Read the model definition and answer for the solid it produces. Units are mm, in the model's axes. A direction names the side the tool comes from. Give positions to 0.01 mm unless a question says otherwise; leave off trailing zeros. Write each loop counter-clockwise with the first axis right and the second up, starting at its lowest first coordinate (ties: lowest second). Pieces come first, ordered by that corner, then holes. Notation, with made-up numbers: (43, -1.5) -> (97, -1.5) arc R14 ccw to (97, 4.5) -> close; hole circle Ø8 at (-32.5, -28). An arc over 180 degrees is marked (long way). Put each result on its own line as item: value. Start each with the question number.
from build123d import *

# Parameters (mm, degrees)
PAD002_DEPTH = 12
PAD_DEPTH    = 2
ARRAY_COUNT  = 3


with BuildPart() as pad002:
    # Sketch002 → Pad002 (new body)
    with BuildSketch(Plane.XY):
        Polygon((-6.6395280957, 11.5), (-7.7942286341, 13.5), (-68, 13.5), (-68, -13.5), (-7.7942286341, -13.5), (-6.6395280957, -11.5), (-66, -11.5), (-66, 11.5), align=None)
    extrude(amount=PAD002_DEPTH)


with BuildPart() as array:
    # Sketch → Pad (new body)
    with BuildSketch(Plane.XY):
        Polygon((0, 0), (-7.7942286341, 13.5), (-68, 13.5), (-68, -13.5), (-7.7942286341, -13.5), align=None)
    extrude(amount=PAD_DEPTH)

    # Fusion: union Pad002
    add(pad002.part)

    # Array: Array ×3 about axis
    array_axis = Axis((0, 0, 0), (0, 0, 1))


with BuildPart() as array_1:
    add(array.part)
    for i in range(1, ARRAY_COUNT):
        add(array.part.rotate(array_axis, i * 360 / ARRAY_COUNT))


solid = array_1.part
1) Straight lines are drawn through the part: line 1 (Y direction, x = 16, z = 8.25); line 2 (Y direction, x = -28, z = 9.25); line 3 (Z direction, x = -63, y = 5). For each, find the intervals that lie inside material, in ascending order. Write a range as [from, to].
2) For faces 4 (the face through (30.429, 25.705, 5.916)), 5 (the face through (0, -1, 0)), 6 (the face through (-37, 11.5, 7)), 7 (the face through (-37, 13.5, 6)), 8 (the face through (-38, -13.5, 6)), determine the directions among +Z, -Z, +X, -X, +Y, -Y from which every point of the face is accessible in a straight line to the end or side of a thin tool.
3) For a pull along Y with two mould halves and no side action, classify faces 1 (the face through (7.468, 39.935, 5.916)), 2 (the face through (-7, -12, 12)), 3 (the face through (-36, -11.5, 7)) as pulls with the +Y half, pulls with the -Y half, needs draft (parallel to the pull), parting line crosses it, or undercut.
4) A cutting plane is placed at C-C on y = -54. Give the vertices of the cut face in (x, z), and give its area (3 significant figures).
5) A cutting plane is placed at A-A on z = 3.5. Give the vertices of the cut face in (x, y).
6) Each of these flat-tipped pins is pushed along its axis until it touches: pin 1 Ø6 at (x, z) = (22, 7) entering from +Y; pin 2 Ø3 at (x, z) = (-49, 8) entering from -Y; pin 3 Ø4 at (y, z) = (-48.5, 5) entering from +X. Where does it stop, or does it pass through?
7) A cutting plane is placed at D-D on x = -21. Give the vertices of the cut face in (y, z), and give its area (3 significant figures).
8) A cutting plane is placed at B-B on x = 38. Give the vertices of the cut face in (y, z), and give its area (3 significant figures).
Results found:
1. line 1: y = [-54.71, -50.71], [-4.71, -0.71], [0.71, 4.71], [50.71, 54.71]
1. line 2: y = [-13.5, -11.5], [11.5, 13.5]
1. line 3: z = [0, 2]
2. face 4: +Z, -Z, +X
2. face 5: -Z, +X, -X, +Y, -Y
2. face 6: +Z
2. face 7: +Z, -Z, -X, +Y
2. face 8: +Z, -Z, -X, -Y
3. face 1: pulls with the +Y half
3. face 2: needs draft
3. face 3: undercut
4. outline: (15.59, 0) -> (42.47, 0) -> (42.47, 12) -> (38.47, 12) -> (38.47, 2) -> (17.9, 2) -> (17.9, 12) -> (15.59, 12) -> close
4. area: 117 mm²
5. outline: (-68, -13.5) -> (-7.79, -13.5) -> (22.31, -65.64) -> (45.69, -52.14) -> (15.59, 0) -> (45.69, 52.14) -> (22.31, 65.64) -> (-7.79, 13.5) -> (-68, 13.5) -> close; hole (-66, -11.5) -> (-6.64, -11.5) -> (23.04, -62.91) -> (42.96, -51.41) -> (13.28, 0) -> (42.96, 51.41) -> (23.04, 62.91) -> (-6.64, 11.5) -> (-66, 11.5) -> close
6. pin 1: stops at y = 65.64
6. pin 2: stops at y = -13.5
6. pin 3: stops at x = 44.74
7. outline: (-13.5, 0) -> (13.5, 0) -> (13.5, 12) -> (11.5, 12) -> (11.5, 2) -> (-11.5, 2) -> (-11.5, 12) -> (-13.5, 12) -> close
7. area: 94.0 mm²
8. outline: (-56.58, 0) -> (-38.82, 0) -> (-38.82, 12) -> (-42.82, 12) -> (-42.82, 2) -> (-54.27, 2) -> (-54.27, 12) -> (-56.58, 12) -> close; (38.82, 0) -> (56.58, 0) -> (56.58, 12) -> (54.27, 12) -> (54.27, 2) -> (42.82, 2) -> (42.82, 12) -> (38.82, 12) -> close
8. area: 197 mm²
